from build123d import *

# Parameters (mm, degrees)
SKETCH_1_R      = 5
SKETCH_1_R_2    = 1.8
EXTRUDE_1_DEPTH = 3
SKETCH_3_R      = 4
SKETCH_3_R_2    = 1.6
EXTRUDE_2_DEPTH = 3


with BuildPart() as part:
    # 草图1 → 凸台-拉伸1 (new body)
    with BuildSketch(Plane.XY):
        with BuildLine():
            Line((5, 0), (21.5, 0))
            ThreePointArc((21.5, 0), (25.035533906, 1.464466094), (26.5, 5))
            Line((26.5, 5), (26.5, 30))
            Line((26.5, 30), (0, 30))
            Line((0, 30), (0, 5))
            ThreePointArc((0, 5), (1.464466094, 1.464466094), (5, 0))
        make_face()
        with Locations((13.25, 15)):
            Circle(SKETCH_1_R, mode=Mode.SUBTRACT)
        with Locations((5.25, 8)):
            Circle(SKETCH_1_R_2, mode=Mode.SUBTRACT)
        with Locations((5.25, 22)):
            Circle(SKETCH_1_R_2, mode=Mode.SUBTRACT)
        with Locations((21.25, 8)):
            Circle(SKETCH_1_R_2, mode=Mode.SUBTRACT)
        with Locations((21.25, 22)):
            Circle(SKETCH_1_R_2, mode=Mode.SUBTRACT)
    extrude(amount=EXTRUDE_1_DEPTH)

    # 草图3 → 凸台-拉伸2 (add)
    with BuildSketch(Plane(origin=(0, 30, 0), x_dir=(1, 0, 0), z_dir=(0, 1, 0))):
        with BuildLine():
            Line((0, -3), (26.5, -3))
            Line((26.5, -3), (26.5, 16.75))
            ThreePointArc((26.5, 16.75), (13.25, 30), (0, 16.75))
            Line((0, 16.75), (0, -3))
        make_face()
        with Locations((13.25, 16.75)):
            Circle(SKETCH_3_R, mode=Mode.SUBTRACT)
        with Locations((21.75, 16.75)):
            Circle(SKETCH_3_R_2, mode=Mode.SUBTRACT)
        with Locations((4.75, 16.75)):
            Circle(SKETCH_3_R_2, mode=Mode.SUBTRACT)
    extrude(amount=EXTRUDE_2_DEPTH)


solid = part.part
CAD build for the part. Positions are in the model's coordinates, mm. A direction names the side the tool comes from. Round coordinates to 2 decimals unless told otherwise and drop trailing zeros. Write each loop counter-clockwise with the first axis right and the second up, starting at its lowest first coordinate (ties: lowest second). Pieces come first, ordered by that corner, then holes.
(1) Slice it at A-A, the plane y = 15. Write the cut outline in (x, z), and give its area (3 significant figures).
(2) Slice it at D-D, the plane z = -16. Write the cut outline in (x, y).
(3) Probe line 1 along Y through (x, z) = (5.25, 1.4); line 2 along X through (y, z) = (30.7, -16.75); line 3 along X through (y, z) = (31, -16). List the from-to ranges inside material, lowest first.
(4) Slice it at C-C, the plane y = 8. Write the cut outline in (x, z), and give its area (3 significant figures).
(5) Drop flat-ended pins along their axis: P1, Ø12, axis at y = 25, z = -20.5, coming from the +X side; P2, Ø6, axis at x = 5.25, y = 22, coming from the +Z side; P3, Ø3, axis at x = 8, y = 16.5, coming from the -Z side; P4, Ø8, axis at x = 9.5, z = -14, coming from the -Y side. Give the stop position or say it passes through.
(6) 3-axis set-ups, long thin cutter, end or side, ignore diameter. For faces 4 (the face through (7, 15, 0)), 5 (the face through (13, 0, 1)): which of +Z, -Z, +X, -X, +Y, -Y reach the whole face in a straight line?
(7) Mould opens along Z. For faces 1 (the face through (16, 20, 3)), 2 (the face through (1, 2, 1)), 3 (the face through (21.542, 31.479, -18.336)) say: pulls with the +Z half, pulls with the -Z half, needs draft (parallel to the pull), parting line crosses it, or undercut.
(8) Slice it at B-B, the plane x = 13.25. Write the cut outline in (y, z).
From the geometry:
1. outline: (0, 0) - (8.25, 0) - (8.25, 3) - (0, 3) - close; (18.25, 0) - (26.5, 0) - (26.5, 3) - (18.25, 3) - close
1. area: 49.5 mm2
2. outline: (0, 30) - (3.34, 30) - (3.34, 33) - (0, 33) - close; (6.16, 30) - (9.32, 30) - (9.32, 33) - (6.16, 33) - close; (17.18, 30) - (20.34, 30) - (20.34, 33) - (17.18, 33) - close; (23.16, 30) - (26.5, 30) - (26.5, 33) - (23.16, 33) - close
3. line 1: y = 0 to 6.2, 9.8 to 20.2, 23.8 to 33
3. line 2: x = 0 to 3.15, 6.35 to 9.25, 17.25 to 20.15, 23.35 to 26.5
3. line 3: x = 0 to 3.34, 6.16 to 9.32, 17.18 to 20.34, 23.16 to 26.5
4. outline: (0, 0) - (3.45, 0) - (3.45, 3) - (0, 3) - close; (7.05, 0) - (19.45, 0) - (19.45, 3) - (7.05, 3) - close; (23.05, 0) - (26.5, 0) - (26.5, 3) - (23.05, 3) - close
4. area: 57.9 mm2
5. P1: stops at x = 26.49
5. P2: stops at z = 3
5. P3: stops at z = 0
5. P4: stops at y = 30
6. face 4: -Z, +X, -X, -Y
6. face 5: +Z, -Z, +X, -X, -Y
7. face 1: pulls with the +Z half
7. face 2: needs draft
7. face 3: undercut
8. outline: (0, 0) - (10, 0) - (10, 3) - (0, 3) - close; (20, 0) - (30, 0) - (30, -12.75) - (33, -12.75) - (33, 3) - (20, 3) - close; (30, -30) - (33, -30) - (33, -20.75) - (30, -20.75) - close
